from build123d import *

# Parameters (mm, degrees)
SKETCH1_W           = 56
SKETCH1_H           = 70
BOSS_EXTRUDE1_DEPTH = 4
SKETCH2_R           = 2.5
SKETCH2_R_2         = 4
SKETCH2_R_3         = 1.6
CUT_EXTRUDE1_DEPTH  = 46.530209751
FILLET1_R           = 3


with BuildPart() as part:
    # Sketch1 → Boss-Extrude1 (new, symmetric)
    with BuildSketch(Plane.XY):
        Rectangle(SKETCH1_W, SKETCH1_H)
    extrude(amount=BOSS_EXTRUDE1_DEPTH, both=True)

    # Sketch2 → Cut-Extrude1 (cut, through all)
    with BuildSketch(Plane.XY.offset(4)):
        with Locations((-23.5, 30.5)):
            Circle(SKETCH2_R)
        with Locations((23.5, 30.5)):
            Circle(SKETCH2_R)
        with Locations((23.5, -16.5)):
            Circle(SKETCH2_R)
        with Locations((-23.5, -16.5)):
            Circle(SKETCH2_R)
        with Locations((0, 7)):
            Circle(SKETCH2_R_2)
        with Locations((-15.5, 22.5)):
            Circle(SKETCH2_R_3)
        with Locations((15.5, 22.5)):
            Circle(SKETCH2_R_3)
        with Locations((15.5, -8.5)):
            Circle(SKETCH2_R_3)
        with Locations((-15.5, -8.5)):
            Circle(SKETCH2_R_3)
    extrude(amount=-CUT_EXTRUDE1_DEPTH, mode=Mode.SUBTRACT)

    # Fillet1
    fillet1_edges = [part.edges().sort_by_distance(p)[0] for p in [
        (28, -35, 0),
        (-28, -35, 0),
        (-28, 35, 0),
        (28, 35, 0),
    ]]
    fillet(fillet1_edges, radius=FILLET1_R)


solid = part.part
Work out the finished part from the listing and answer in its coordinate system (mm). Round coordinates to 2 decimals unless told otherwise and drop trailing zeros. Write each loop counter-clockwise with the first axis right and the second up, starting at its lowest first coordinate (ties: lowest second). Pieces come first, ordered by that corner, then holes. Notation, with made-up numbers: (-37.5, -16.5) -> (2.5, -16.5) arc R15 ccw to (2.5, -5.5) -> close; hole circle Ø2 at (-34.75, -21.75). An arc over 180 degrees is marked (long way). Write each question's results on one line, items separated by ' | '.
Item 1: Flat-ended cylindrical pins translate along their axes: P1, Ø4, axis at x = 15.5, y = 22.5, coming from the -Z side; P2, Ø4.5, axis at x = -23.5, y = -16.5, coming from the +Z side. Find the tip coordinate at first contact, or state that the pin passes through.
Result set:
P1: z = -4 | P2: through
Item 2: A cutting plane is placed at A-A, the plane x = 0. Determine the outline of the cut face in (y, z).
Result set:
outline: (-35, -4) -> (3, -4) -> (3, 4) -> (-35, 4) -> close; (11, -4) -> (35, -4) -> (35, 4) -> (11, 4) -> close
Item 3: A cutting plane is placed at D-D, the plane y = 7. Determine the outline of the cut face in (x, z).
Result set:
outline: (-28, -4) -> (-4, -4) -> (-4, 4) -> (-28, 4) -> close; (4, -4) -> (28, -4) -> (28, 4) -> (4, 4) -> close
Item 4: A cutting plane is placed at C-C, the plane z = 2.25. Count the separate pieces of the cut face and the enclosed holes in it, plus the area to 3 significant figures.
Result set:
separate pieces: 1 | enclosed holes: 9 | area: 3,750 mm^2
Item 5: Find the intervals of material crossed by line 1 along Y through (x, z) = (-15.5, 0.5); line 2 along Y through (x, z) = (23.5, -0.25); line 3 along X through (y, z) = (-7.5, -1.5), in increasing order. Write a range as [from, to].
Result set:
line 1: [-35, -10.1], [-6.9, 20.9], [24.1, 35] | line 2: [-35, -19], [-14, 28], [33, 35] | line 3: [-28, -16.75], [-14.25, 14.25], [16.75, 28]
Item 6: The mould has two halves that part along X. Classify faces 1 (the face through (-28, 0, 0)), 2 (the face through (-16.68, 23.58, 0.06)), 3 (the face through (0, 0, 4)): +X half, -X half, draft (parallel to the pull), parting line (faces both ways), or undercut.
Result set:
face 1: -X half | face 2: undercut | face 3: draft
Item 7: A cutting plane is placed at B-B, the plane x = 23.5. Determine the outline of the cut face in (y, z), plus the area to 3 significant figures.
Result set:
outline: (-35, -4) -> (-19, -4) -> (-19, 4) -> (-35, 4) -> close; (-14, -4) -> (28, -4) -> (28, 4) -> (-14, 4) -> close; (33, -4) -> (35, -4) -> (35, 4) -> (33, 4) -> close | area: 480 mm^2
